from build123d import *

# Parameters (mm, degrees)
SKETCH_1_W          = 10
SKETCH_1_H          = 10
SKETCH_1_W_2        = 8
SKETCH_1_H_2        = 8
EXTRUDE_1_DEPTH     = 445.586099411
SKETCH_2_R          = 2.1
CUT_EXTRUDE_1_DEPTH = 446.72634204


with BuildPart() as part:
    # ｽｹｯﾁ1 → 押し出し-薄板1 (new body)
    with BuildSketch(Plane(origin=(0, 0, 0), x_dir=(0, -1, 0), z_dir=(1, 0, 0))):
        Rectangle(SKETCH_1_W, SKETCH_1_H)
        Rectangle(SKETCH_1_W_2, SKETCH_1_H_2, mode=Mode.SUBTRACT)
    extrude(amount=EXTRUDE_1_DEPTH)

    # ｽｹｯﾁ2 → ｶｯﾄ - 押し出し1 (cut, through all)
    with BuildSketch(Plane(origin=(0, 5, 0), x_dir=(1, 0, 0), z_dir=(0, 1, 0))):
        with Locations(Location((5, 0, 0), (0, 0, 270))):
            Circle(SKETCH_2_R)
        with Locations(Location((440.586099411, 0, 0), (0, 0, 270))):
            Circle(SKETCH_2_R)
    extrude(amount=-CUT_EXTRUDE_1_DEPTH, mode=Mode.SUBTRACT)


solid = part.part
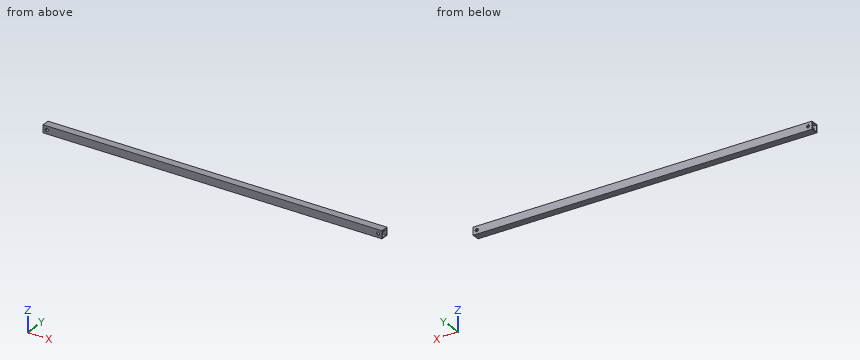
Model file for the job. Use its own axes, mm. Round coordinates to 2 decimals unless told otherwise and drop trailing zeros. Order: outer loops, then holes, each group sorted by start corner. A loop starts at its lowest first (then second) coordinate and runs counter-clockwise, first axis right, second up.
(1) Drill centre lines: line 1 (X direction, y = 4.6, z = 0); line 2 (Z direction, x = 153, y = -2). Where is each one in solid material? Low to high.
(2) Band-saw the part on A-A (y = -0.5). List the corners of the cut face in (x, z), then the cut area to 3 significant figures.
(3) Band-saw the part on B-B (z = 0). List the corners of the cut face in (x, y), then the cut area to 3 significant figures.
(4) Band-saw the part on C-C (x = 52). List the corners of the cut face in (y, z).
(5) Pin check, flat tip, straight feed: pin 1 (4 mm diameter, centred on x = 5, z = 0, fed in from -Y). Stop position of the tip, or through.
Verdict:
1. line 1: x = 0 to 2.9, 7.1 to 438.49, 442.69 to 445.59
1. line 2: z = -5 to -4, 4 to 5
2. outline: (0, -5) - (445.59, -5) - (445.59, -4) - (0, -4) - close; (0, 4) - (445.59, 4) - (445.59, 5) - (0, 5) - close
2. area: 891 mm2
3. outline: (0, -5) - (2.9, -5) - (2.9, -4) - (0, -4) - close; (0, 4) - (2.9, 4) - (2.9, 5) - (0, 5) - close; (7.1, -5) - (438.49, -5) - (438.49, -4) - (7.1, -4) - close; (7.1, 4) - (438.49, 4) - (438.49, 5) - (7.1, 5) - close; (442.69, -5) - (445.59, -5) - (445.59, -4) - (442.69, -4) - close; (442.69, 4) - (445.59, 4) - (445.59, 5) - (442.69, 5) - close
3. area: 874 mm2
4. outline: (-5, -5) - (5, -5) - (5, 5) - (-5, 5) - close; hole (-4, -4) - (4, -4) - (4, 4) - (-4, 4) - close
5. pin 1: passes through
